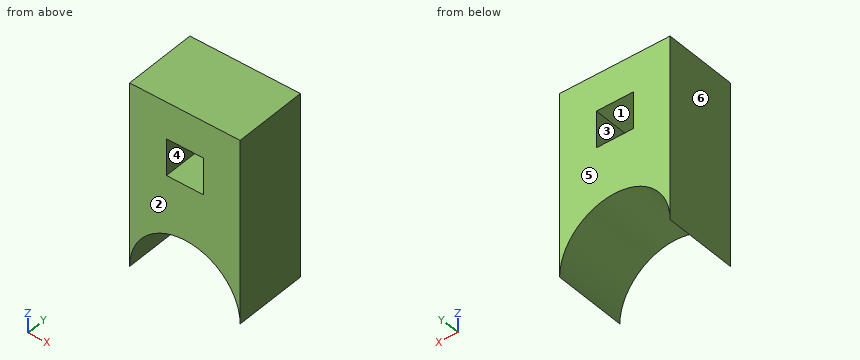
Autodesk Inventor part; units mm, degrees
ref_plane "YZ Plane" through (0, 0, 0) normal (1, 0, 0) x (0, 1, 0)
ref_plane "XZ Plane" through (0, 0, 0) normal (0, 1, 0) x (-1, 0, 0)
ref_plane "XY Plane" through (0, 0, 0) normal (0, 0, 1) x (1, 0, 0)
sketch "スケッチ1" plane through (0, 0, 0) normal (0, 1, 0) x (-1, 0, 0)
  line L0 (8.4764, 10.991) -> (-21.5236, 10.991)
  line L1 (-21.5236, 10.991) -> (-21.5236, -39.009)
  line L2 (-21.5236, -39.009) -> (8.4764, -39.009)
  line L3 (8.4764, -39.009) -> (8.4764, 10.991)
  point P0 (0, 0)
  dimension "d0" = 30
  dimension "d1" = 50
extrude "押し出し1" add sketch "スケッチ1" along normal blind 20
sketch "スケッチ2" plane through (0, 20, 0) normal (0, 1, 0) x (1, 0, 0)
  line L0 (21.5236, 39.009) -> (-8.4764, 39.009)
  circle A0 centre (6.5236, 39.009) radius 15
  point P0 (0, 0)
  dimension "d4" = 30
hole "穴1" at (6.5236, 20, -39.009) direction (0, -1, 0) diameter 30 depth 20
sketch "スケッチ3" plane through (0, 20, 0) normal (0, 1, 0) x (1, 0, 0)
  line L0 (1.5236, -0.991) -> (11.5236, -0.991)
  line L1 (11.5236, -0.991) -> (11.5236, 9.009)
  line L2 (11.5236, 9.009) -> (1.5236, 9.009)
  line L3 (1.5236, 9.009) -> (1.5236, -0.991)
  line L4 (-8.4764, 39.009) -> (-8.4764, -10.991)
  line L5 (-8.4764, -10.991) -> (21.5236, -10.991)
  point P0 (0, 0)
  dimension "d12" = 10
  dimension "d13" = 10
  dimension "d14" = 10
  dimension "d15" = 10
extrude "押し出し2" cut sketch "スケッチ3" against normal blind 20
equation "\"BendRadius\" = Thickness"
equation "\"BendReliefWidth\" = Thickness"
equation "\"BendReliefDepth\" = 0.5 * Thickness"
equation "\"CornerReliefSize\" = 4 * Thickness"
equation "\"MinimumRemnant\" = 2 * Thickness"
equation "\"TransitionRadius\" = BendRadius"
equation "\"JacobiRadiusSize\" = BendRadius"
equation "\"GapSize\" = Thickness"
Check sheet for the modelled part. Datum: model origin and axes. Units: mm. Face numbers are marked on the shaded views. A direction names the side the tool comes from. Give positions to 0.01 mm unless a question says otherwise; leave off trailing zeros. Write each loop counter-clockwise with the first axis right and the second up, starting at its lowest first coordinate (ties: lowest second). Pieces come first, ordered by that corner, then holes. Notation, with made-up numbers: (14.5, 73) - (36.5, 73) arc R11 cw to (36.5, 89) - close; hole circle Ø3 at (-40, -1.75). An arc over 180 degrees is marked (long way). Answer as a JSON object with one key per item and string values. Group by question number.
1) Sectioned sample at D-D (x = -2.75). Record the cut outline in (y, z), then the cut area to 3 significant figures.
2) Access from +Z, -Z, +X, -X, +Y, -Y to the whole of each face (thin tool, end or side, straight path). Record for the marked faces 1 and 2.
3) Release check for a two-part mould opening along X. For the marked faces 3, 4, 5 and 6 record: pulls with the +X half, pulls with the -X half, needs draft (parallel to the pull), parting line crosses it, or undercut.
4) Sectioned sample at A-A (y = 8.5). Record the cut outline in (x, z), then the cut area to 3 significant figures.
5) Sectioned sample at B-B (z = -2.5). Record the cut outline in (x, y), then the cut area to 3 significant figures.
6) Depth check by flat-ended pin: P1, Ø3, axis at x = 17.5, y = 13, coming from the -Z side; P2, Ø8, axis at x = 0.5, y = 18, coming from the -Z side; P3, Ø11, axis at x = 7, y = 7, coming from the -Z side. Enter the tip coordinate at first touch or a pass-through.
7) Sectioned sample at C-C (x = 8.25). Record the cut outline in (y, z), then the cut area to 3 significant figures.
8) Thickness scan on probe 1 along X at (y, z) = (3.75, -1.5); probe 2 along X at (y, z) = (10.25, -33); probe 3 along Z at (x, y) = (8.5, 8). Record the ranges inside material, lowest first. Write a range as from..to.
Geometry results:
{
 "1": {"outline": "(0, -27.22) - (20, -27.22) - (20, 10.99) - (0, 10.99) - close", "area": "764 mm^2"},
 "2": {"face 1": "+Y, -Y", "face 2": "+Z, -Z, +X, -X, -Y"},
 "3": {"face 3": "undercut", "face 4": "undercut", "face 5": "needs draft", "face 6": "pulls with the -X half"},
 "4": {"outline": "(-8.48, -39.01) arc R15 cw to (21.52, -39.01) - (21.52, 10.99) - (-8.48, 10.99) - close; hole (1.52, -9.01) - (11.52, -9.01) - (11.52, 0.99) - (1.52, 0.99) - close", "area": "1,050 mm^2"},
 "5": {"outline": "(-8.48, 0) - (1.52, 0) - (1.52, 20) - (-8.48, 20) - close; (11.52, 0) - (21.52, 0) - (21.52, 20) - (11.52, 20) - close", "area": "400 mm^2"},
 "6": {"P1": "stops at z = -30.68", "P2": "stops at z = -27.85", "P3": "stops at z = -25.25"},
 "7": {"outline": "(0, -24.11) - (20, -24.11) - (20, -9.01) - (0, -9.01) - close; (0, 0.99) - (20, 0.99) - (20, 10.99) - (0, 10.99) - close", "area": "502 mm^2"},
 "8": {"probe 1": "x = -8.48..1.52, 11.52..21.52", "probe 2": "x = -8.48..-7.22, 20.27..21.52", "probe 3": "z = -24.14..-9.01, 0.99..10.99"}
}
